```python
from build123d import *

# Parameters (mm, degrees)
BOSS_EXTRUDE1_DEPTH   = 4.064
BOSS_EXTRUDE1_2_DEPTH = 4.064
SKETCH2_W             = 44.1071
SKETCH2_H             = 24.0792
SKETCH2_R             = 3.81
BOSS_EXTRUDE2_DEPTH   = 2.032
F_3_CLEARANCE_HOLE1_D = 2.794


with BuildPart() as part:
    # Sketch1 → Boss-Extrude1 (new body)
    with BuildSketch(Plane.XY):
        with BuildLine():
            Line((-22.05355, -18.6229), (-22.05355, -12.2729))
            ThreePointArc((-22.05355, -12.2729), (-20.193678061, -7.782771939), (-15.70355, -5.9229))
            Line((-15.70355, -5.9229), (15.70355, -5.9229))
            ThreePointArc((15.70355, -5.9229), (20.193678061, -7.782771939), (22.05355, -12.2729))
            Line((22.05355, -12.2729), (22.05355, -18.6229))
            Line((22.05355, -18.6229), (-22.05355, -18.6229))
        make_face()
    extrude(amount=BOSS_EXTRUDE1_DEPTH)



with BuildPart() as body_2:
    # Sketch1 → Boss-Extrude1 2 (new body)
    with BuildSketch(Plane.XY):
        with BuildLine():
            Line((-22.05355, -36.3521), (22.05355, -36.3521))
            Line((22.05355, -36.3521), (22.05355, -42.7021))
            ThreePointArc((22.05355, -42.7021), (20.193678061, -47.192228061), (15.70355, -49.0521))
            Line((15.70355, -49.0521), (-15.70355, -49.0521))
            ThreePointArc((-15.70355, -49.0521), (-20.193678061, -47.192228061), (-22.05355, -42.7021))
            Line((-22.05355, -42.7021), (-22.05355, -36.3521))
        make_face()
    extrude(amount=BOSS_EXTRUDE1_2_DEPTH)


with BuildPart() as part_1:
    add(part.part)

    add(body_2.part)  # Boss-Extrude2 merges body 2
    # Sketch2 → Boss-Extrude2 (add)
    with BuildSketch(Plane.XY.offset(4.064)):
        with Locations((0, -27.4875)):
            Rectangle(SKETCH2_W, SKETCH2_H)
        with Locations((14.43355, -27.4875)):
            Circle(SKETCH2_R, mode=Mode.SUBTRACT)
        with Locations((-14.43355, -27.4875)):
            Circle(SKETCH2_R, mode=Mode.SUBTRACT)
        Polygon((-6.77545, -23.77275), (-6.77545, -24.71255), (-6.77545, -30.26245), (-6.77545, -31.20225), (6.77545, -31.20225), (6.77545, -23.77275), align=None, mode=Mode.SUBTRACT)
    extrude(amount=-BOSS_EXTRUDE2_DEPTH)

    # #3 Clearance Hole1 (through all)
    with Locations(Plane.XY.offset(4.064)):
        with Locations((0, -10.6854), (0, -44.2896)):
            Hole(F_3_CLEARANCE_HOLE1_D / 2)


solid = part_1.part
```
Could you check a few things on this model? Use its own coordinates, in mm. A direction names the side the tool comes from. Coordinates: 2 decimals unless noted, no trailing zeros. Write each loop counter-clockwise with the first axis right and the second up, starting at its lowest first coordinate (ties: lowest second). Pieces come first, ordered by that corner, then holes. Notation, with made-up numbers: (75, -34) - (102, -34) arc R23 cw to (102, -26) - close; hole circle Ø8 at (-18.5, 19). An arc over 180 degrees is marked (long way). Use a Markdown table: item, result.
Q1. Thinking about a two-plate mould opening in Y: for faces 4 (the cylindrical face through (-10.8, -26.34, 3.06)), 5 (the cylindrical face through (-20.144, -47.241, 2.004)), 6 (the cylindrical face through (-20.24, -7.83, 2)), which applies, +Y half, -Y half, draft (parallel to the pull), parting line (faces both ways), or undercut?
Geometry check:
| item | result |
|---|---|
| face 4 | undercut |
| face 5 | -Y half |
| face 6 | +Y half |
Q2. Imagine slicing it at C-C (z = 1.4). List the corners of the cut face in (x, y) for me.
Geometry check:
| item | result |
|---|---|
| outline | (-22.05, -42.7) arc R6.35 ccw to (-15.7, -49.05) - (15.7, -49.05) arc R6.35 ccw to (22.05, -42.7) - (22.05, -36.35) - (-22.05, -36.35) - close; (-22.05, -18.62) - (22.05, -18.62) - (22.05, -12.27) arc R6.35 ccw to (15.7, -5.92) - (-15.7, -5.92) arc R6.35 ccw to (-22.05, -12.27) - close; hole circle Ø2.79 at (0, -44.29); hole circle Ø2.79 at (0, -10.69) |
Q3. Please list where these lines run through material, in increasing order: L1, parallel to Y at x = 0, z = 1.6; L2, parallel to Y at x = 0, z = 3.1; L3, parallel to Y at x = -14.5, z = 3.5.
Geometry check:
| item | result |
|---|---|
| L1 | y = -49.05 to -45.69, -42.89 to -36.35, -18.62 to -12.08, -9.29 to -5.92 |
| L2 | y = -49.05 to -45.69, -42.89 to -31.2, -23.77 to -12.08, -9.29 to -5.92 |
| L3 | y = -49.05 to -31.3, -23.68 to -5.92 |
Q4. Imagine slicing it at D-D (y = -45). List the corners of the cut face in (x, z) for me.
Geometry check:
| item | result |
|---|---|
| outline | (-21.62, 0) - (-1.2, 0) - (-1.2, 4.06) - (-21.62, 4.06) - close; (1.2, 0) - (21.62, 0) - (21.62, 4.06) - (1.2, 4.06) - close |
Q5. Imagine slicing it at B-B (x = 0). List the corners of the cut face in (y, z) for me.
Geometry check:
| item | result |
|---|---|
| outline | (-49.05, 0) - (-45.69, 0) - (-45.69, 4.06) - (-49.05, 4.06) - close; (-42.89, 0) - (-36.35, 0) - (-36.35, 2.03) - (-31.2, 2.03) - (-31.2, 4.06) - (-42.89, 4.06) - close; (-23.77, 2.03) - (-18.62, 2.03) - (-18.62, 0) - (-12.08, 0) - (-12.08, 4.06) - (-23.77, 4.06) - close; (-9.29, 0) - (-5.92, 0) - (-5.92, 4.06) - (-9.29, 4.06) - close |
Q6. Imagine slicing it at A-A (x = 5). List the corners of the cut face in (y, z) for me, and give its area (3 significant figures).
Geometry check:
| item | result |
|---|---|
| outline | (-49.05, 0) - (-36.35, 0) - (-36.35, 2.03) - (-31.2, 2.03) - (-31.2, 4.06) - (-49.05, 4.06) - close; (-23.77, 2.03) - (-18.62, 2.03) - (-18.62, 0) - (-5.92, 0) - (-5.92, 4.06) - (-23.77, 4.06) - close |
| area | 124 mm2 |
Q7. I'm going to push flat-ended pins straight in: pin 1 Ø9 at (x, y) = (14.43, -27.49) entering from -Z; pin 2 Ø1.7 at (x, y) = (0, -44.29) entering from +Z. Where does each tip first touch, or does it pass through?
Geometry check:
| item | result |
|---|---|
| pin 1 | stops at z = 2.03 |
| pin 2 | passes through |
Q8. Which directions (+Z, -Z, +X, -X, +Y, -Y) give clear straight access to the entire face, cutting with the end or side of a thin tool? Please do faces 1 (the flat face through (22.054, -27.3, 2.5)), 2 (the flat face through (0, -36.352, 1)), 3 (the flat face through (0, -23.773, 3)).
Geometry check:
| item | result |
|---|---|
| face 1 | +Z, -Z, +X, +Y, -Y |
| face 2 | -Z, +X, -X |
| face 3 | +Z, -Z |
